The model under review builds one solid part; all positions refer to its coordinate system, in mm. Face numbers are marked on the shaded views. Coordinates: 2 decimals unless noted, no trailing zeros. Write each loop counter-clockwise with the first axis right and the second up, starting at its lowest first coordinate (ties: lowest second). Pieces come first, ordered by that corner, then holes. Notation, with made-up numbers: (9.5, 79.5) -> (48.5, 79.5) arc R26 ccw to (48.5, 102.5) -> close; hole circle Ø5 at (30.25, 36). An arc over 180 degrees is marked (long way). Write each question's results on one line, items separated by ' | '.
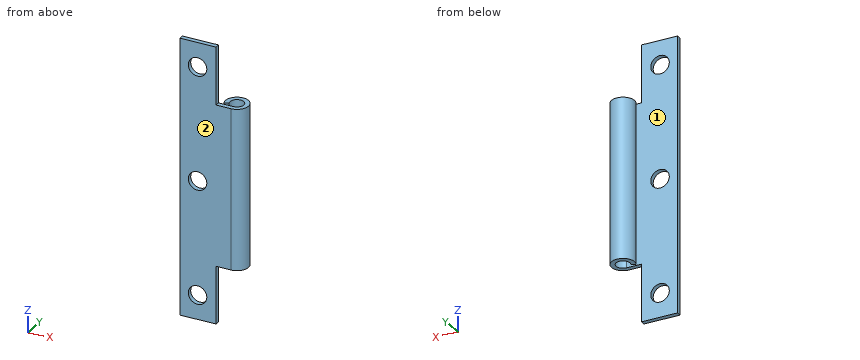
```python
from build123d import *

# Parameters (mm, degrees)
SKETCH3_W          = 60
SKETCH3_H          = 1
SKETCH4_W          = 8.09810269
SKETCH4_H          = 14.216859333
SKETCH4_W_2        = 8.260259714
SKETCH4_H_2        = 13.467623065
CUT_EXTRUDE1_DEPTH = 62.702917273
SKETCH5_R          = 2
CUT_EXTRUDE2_DEPTH = 62.629944021


with BuildPart() as part:
    # Sweep1: sweep along a path in Sketch1
    with BuildLine(Plane.XY) as sweep1_path:
        Line((0, 0), (11, 0))
        ThreePointArc((11, 0), (12.315747679, 4.62574882), (8.762440739, 1.384953564))
    # Sketch3 → Sweep1 (sweep)
    with BuildSketch(Plane(origin=(0, 0, 0), x_dir=(0, 0, -1), z_dir=(1, 0, 0))):
        with Locations((-30, 0.5)):
            Rectangle(SKETCH3_W, SKETCH3_H)
    sweep(path=sweep1_path.line)

    # Sketch4 → Cut-Extrude1 (cut, through all)
    with BuildSketch(Plane(origin=(0, 0, 0), x_dir=(-1, 0, 0), z_dir=(0, -1, 0))):
        with Locations((-11.830088217, -54.549659974)):
            Rectangle(SKETCH4_W, SKETCH4_H)
        with Locations((-11.911166729, -5.766188468)):
            Rectangle(SKETCH4_W_2, SKETCH4_H_2)
    extrude(amount=-CUT_EXTRUDE1_DEPTH, mode=Mode.SUBTRACT)

    # Sketch5 → Cut-Extrude2 (cut, through all)
    with BuildSketch(Plane(origin=(0, 1, 0), x_dir=(1, 0, 0), z_dir=(0, 1, 0))):
        with Locations(Location((3.794583691, -5.285866517, 0), (0, 0, 270))):
            Circle(SKETCH5_R)
        with Locations(Location((3.794583691, -54.714133483, 0), (0, 0, 90))):
            Circle(SKETCH5_R)
        with Locations(Location((3.794583691, -30, 0), (0, 0, 270))):
            Circle(SKETCH5_R)
    extrude(amount=-CUT_EXTRUDE2_DEPTH, mode=Mode.SUBTRACT)


solid = part.part
```
Q1. Clearance check with flat-ended pins moving along their axes: P1, Ø2, axis at x = 6, y = 3.5, coming from the -Z side; P2, Ø2, axis at y = 1.5, z = 37.5, coming from the +X side; P3, Ø1.1, axis at y = 0.5, z = 51, coming from the +X side; P4, Ø2.5, axis at x = 12, y = 2, coming from the +Z side. State where each tip first meets the part, or that it passes through.
Solution:
P1: through | P2: x = 13.5 | P3: x = 7.78 | P4: z = 47.44
Q2. Add section B-B (z = 30). Write out the cut boundary in (x, y).
Solution:
outline: (0, 0) -> (1.79, 0) -> (1.79, 1) -> (0, 1) -> close; (5.79, 0) -> (11, 0) arc R2.5 ccw (long way) to (8.76, 1.38) -> (9.66, 1.83) arc R1.5 cw (long way) to (11, 1) -> (5.79, 1) -> close
Q3. Add section C-C (z = 14). Write out the cut boundary in (x, y), plus the area to 3 significant figures.
Solution:
outline: (0, 0) -> (11, 0) arc R2.5 ccw (long way) to (8.76, 1.38) -> (9.66, 1.83) arc R1.5 cw (long way) to (11, 1) -> (0, 1) -> close | area: 21.3 mm²
Q4. Add section A-A (y = 2.5). Write out the cut boundary in (x, z).
Solution:
outline: (8.5, 12.5) -> (9.5, 12.5) -> (9.5, 47.44) -> (8.5, 47.44) -> close; (12.5, 12.5) -> (13.5, 12.5) -> (13.5, 47.44) -> (12.5, 47.44) -> close
Q5. Draft analysis for pull direction Y (two halves, no side actions). For the marked faces 1 and 2, state which applies: pulls with the +Y half, pulls with the -Y half, needs draft (parallel to the pull), parting line crosses it, or undercut.
Solution:
face 1: undercut | face 2: pulls with the -Y half
Q6. For line 1 (Y direction, x = 11, z = 27); line 2 (Z direction, x = 11.25, y = 4.1); line 3 (Y direction, x = 2.5, z = 35), list the stretches that pass through material, from the lowest coordinate up. Write a range as from..to.
Solution:
line 1: 0..1, 4..5 | line 2: 12.5..47.44 | line 3: 0..1
